Autodesk Inventor part; units mm, degrees
ref_plane "YZ Plane" through (0, 0, 0) normal (1, 0, 0) x (0, 1, 0)
ref_plane "XZ Plane" through (0, 0, 0) normal (0, 1, 0) x (-1, 0, 0)
ref_plane "XY Plane" through (0, 0, 0) normal (0, 0, 1) x (1, 0, 0)
sketch "Sketch1" plane through (0, 0, 0) normal (0, 0, 1) x (1, 0, 0)
  line L0 (-4.5901, 0) -> (-2.295, 3.9751)
  line L1 (-2.295, 3.9751) -> (2.295, 3.9751)
  line L2 (2.295, 3.9751) -> (4.5901, 0)
  line L3 (4.5901, 0) -> (2.295, -3.9751)
  line L4 (2.295, -3.9751) -> (-2.295, -3.9751)
  line L5 (-2.295, -3.9751) -> (-4.5901, 0)
  point P0 (0, 0)
  dimension "d2" = 7.9502
extrude "Extrusion1" add sketch "Sketch1" along normal blind 3.9878
sketch "Sketch2" plane through (0, 0, 3.9878) normal (0, 0, 1) x (1, 0, 0)
  circle A0 centre (0, 0) radius 3.556
  dimension "d5" = 7.112
extrude "Extrusion2" add sketch "Sketch2" along normal blind 1.27
sketch "Sketch3" plane through (0, 0, 5.2578) normal (0, 0, 1) x (1, 0, 0)
  circle A0 centre (0, 0) radius 3.556
  circle A1 centre (0, 0.7874) radius 2.1
  dimension "d10" = 4.2
  dimension "d11" = 0.7874
hole "Hole1" at (0, 0.7874, 5.2578) direction (0, 0, -1) diameter 4.1402 end through all
chamfer "Chamfer1" distance 0.254 angle 45 6 edges at (3.4425, -1.9875, 0) (3.4425, 1.9876, 0) (0, 3.9751, 0) (-3.4425, 1.9875, 0) (-3.4425, -1.9876, 0) (0, -3.9751, 0)
properties part number "B18033" material "Stainless Steel"
For this review, take the finished solid that the model builds, in its own axes (mm). A direction names the side the tool comes from. Give positions to 0.01 mm unless a question says otherwise; leave off trailing zeros. Loops run counter-clockwise (first coordinate to the right, second up) from the corner with the lowest first, then second, coordinate; pieces in that order, holes last. Notation, with made-up numbers: M -4.5,-36 L 15.5,-36 A22 cw 15.5,-14 Z; hole C 51,74 d8. An arc over 180 degrees is marked long. Put each result on its own line as item: value. Start each with the question number.
(1) The part is to be moulded in two halves that separate along Y. For faces 1 (the flat face through (0, 3.975, 2)), 2 (the flat face through (3.46, -1.96, 2.09)), 3 (the flat face through (1.7, 3.3, 3.988)), 4 (the cylindrical face through (-1.4, 2.31, 2.59)), say which applies: +Y half, -Y half, draft (parallel to the pull), parting line (faces both ways), or undercut.
(2) Add section A-A, the plane z = 2.15. Write out the cut boundary in (x, y) (3 decimals), then the cut area to 3 significant figures.
(3) Wall thickness on L1, parallel to Y at x = 0, z = 2.65; L2, parallel to Z at x = 2, y = 3.25; L3, parallel to Y at x = 0, z = 4.1: over which ranges is each line inside the solid? List them lowest first.
(4) Add section D-D, the plane y = -3. Write out the cut boundary in (x, z).
(5) Add section B-B, the plane x = 0. Write out the cut boundary in (y, z).
(6) Add section C-C, the plane y = 1.5. Write out the cut boundary in (x, z), then the cut area to 3 significant figures.
(7) Machinability: for faces 5 (the flat face through (-3.46, 1.96, 2.09)), 6 (the cylindrical face through (-0.77, 3.47, 4.61)), which of the approach directions +Z, -Z, +X, -X, +Y, -Y give a long, thin tool a straight path to every point of the face, cutting with its end or side? Answer none if there is none.
(8) For pin 1 (1.5 mm diameter, centred on y = 3, z = 1, fed in from +X); pin 2 (2.5 mm diameter, centred on x = 0, y = 0.79, fed in from +Z); pin 3 (4 mm diameter, centred on x = -3.5, y = 1.5, fed in from -Z), all flat-tipped, find the tip position at first contact; note any pin that passes through.
Result:
1. face 1: +Y half
1. face 2: -Y half
1. face 3: draft
1. face 4: undercut
2. outline: M -4.59,0 L -2.295,-3.975 L 2.295,-3.975 L 4.59,0 L 2.295,3.975 L -2.295,3.975 Z; hole C 0,0.787 d4.14
2. area: 41.3 mm^2
3. L1: y = -3.98 to -1.28, 2.86 to 3.98
3. L2: z = 0 to 3.99
3. L3: y = -3.56 to -1.28, 2.86 to 3.56
4. outline: M -2.86,0.25 L -2.56,0 L 2.56,0 L 2.86,0.25 L 2.86,3.99 L 1.91,3.99 L 1.91,5.26 L -1.91,5.26 L -1.91,3.99 L -2.86,3.99 Z
5. outline: M -3.98,0.25 L -3.72,0 L -1.28,0 L -1.28,5.26 L -3.56,5.26 L -3.56,3.99 L -3.98,3.99 Z; M 2.86,0 L 3.72,0 L 3.98,0.25 L 3.98,3.99 L 3.56,3.99 L 3.56,5.26 L 2.86,5.26 Z
6. outline: M -3.72,0.25 L -3.43,0 L -1.94,0 L -1.94,5.26 L -3.22,5.26 L -3.22,3.99 L -3.72,3.99 Z; M 1.94,0 L 3.43,0 L 3.72,0.25 L 3.72,3.99 L 3.22,3.99 L 3.22,5.26 L 1.94,5.26 Z
6. area: 17.4 mm^2
7. face 5: +Z, -Z, -X, +Y
7. face 6: +Z
8. pin 1: stops at x = 3.29
8. pin 2: passes through
8. pin 3: stops at z = 0
